Source: three-view drawing plus pictorial views. Frame: mm from the lowest corner of the part. A direction names the side the tool comes from. Coordinates: 2 decimals unless noted, no trailing zeros. Write each loop counter-clockwise with the first axis right and the second up, starting at its lowest first coordinate (ties: lowest second). Pieces come first, ordered by that corner, then holes. Notation, with made-up numbers: (52, 77) - (69, 77) arc R33 ccw to (69, 112) - close; hole circle Ø6 at (37, -10). An arc over 180 degrees is marked (long way). One line per item, written item: value.
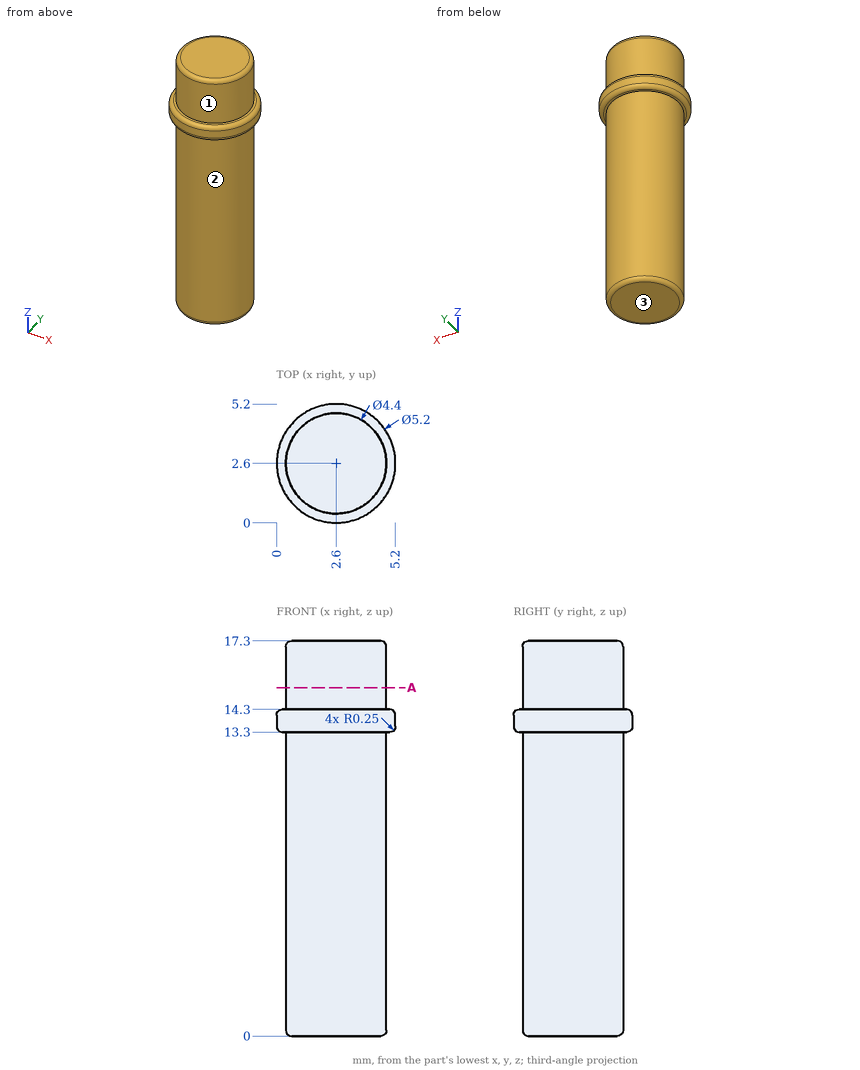
1) Reachability of the marked faces 1, 2 and 3 from +Z, -Z, +X, -X, +Y, -Y: full face, straight path, thin tool, end or side. Return the list, or none.
Values found:
face 1: +Z
face 2: -Z
face 3: -Z, +X, -X, +Y, -Y
2) Section query A-A on z = 15.25. Output: boundary loops of the cut face in (x, y), then the cut area to 3 significant figures.
Values found:
outline: circle Ø4.4 at (2.6, 2.6)
area: 15.2 mm2
3) Material intervals for line 1 (Y direction, x = 2.5, z = 11); line 2 (Z direction, x = 4.4, y = 4); line 3 (X direction, y = 2.25, z = 1.75), sorted ascending.
Values found:
line 1: 0.4 to 4.8
line 2: 13.3 to 14.3
line 3: 0.43 to 4.77
4) Contact query for flat-ended pins moving along their axis: P1, Ø2, axis at y = 3, z = 1.5, coming from the -X side; P2, Ø1.5, axis at x = 4.5, z = 15.5, coming from the -Y side; P3, Ø2, axis at x = 1, z = 3.5, coming from the -Y side. Output: stop coordinate, or through.
Values found:
P1: x = 0.4
P2: y = 0.72
P3: y = 0.48
